Verification items for the finished model (mm, model axes). A direction names the side the tool comes from. Coordinates: 2 decimals unless noted, no trailing zeros. Order: outer loops, then holes, each group sorted by start corner. A loop starts at its lowest first (then second) coordinate and runs counter-clockwise, first axis right, second up. Notation, with made-up numbers: M 6.25,42 L 44.25,42 A10 ccw 44.25,57 Z; hole C 48,60.25 d11. An arc over 180 degrees is marked long. Return JSON: item names as keys, results as strings. Group by question number.
Q1. Thickness scan on probe 1 along Z at (x, y) = (-0.95, 0); probe 2 along X at (y, z) = (0.15, 30); probe 3 along Y at (x, z) = (-0.95, 3). Record the ranges inside material, lowest first.
Q2. Section check C-C, the plane z = 3. Enter the section's corners in (x, y), then the cut area to 3 significant figures.
Q3. Section check A-A, the plane y = 0. Enter the section's corners in (x, z), then the cut area to 4 significant figures.
Q4. Mould release check, pull along X, two halves, no side actions. Record for faces 3 (the face through (-0.5, 0, 5)), 4 (the face through (-2, 0, 20)), 5 (the face through (1.4, 0, 0.4)): pulls with the +X half, pulls with the -X half, needs draft (parallel to the pull), parting line crosses it, or undercut.
Q5. Go/stop test with flat-tipped pins: pin 1 Ø0.8 at (x, y) = (0, 0.5) entering from -Z; pin 2 Ø1.8 at (y, z) = (0, 3) entering from +X; pin 3 Ø1.2 at (y, z) = (-0.5, 2.5) entering from -X. Record where each tip stops, or that it passes through.
Q6. Section check D-D, the plane z = 10. Enter the section's corners in (x, y).
Q7. Section check B-B, the plane x = 0. Enter the section's corners in (y, z), then the cut area to 3 significant figures.
Q8. Access from +Z, -Z, +X, -X, +Y, -Y to the whole of each face (thin tool, end or side, straight path). Record for faces 1 (the face through (0.5, 0, 5)), 2 (the face through (-1, 0, 2)).
from build123d import *

# Parameters (mm, degrees)
SKETCH_1_R                 = 2
EXTRUDE_338_DEPTH          = 40
CHAMFER_1_SIZE             = 1
CUT_EXTRUDE_518_DEPTH      = 41.099875312
CUT_EXTRUDE_518_DEPTH_BACK = 41.099875312
SKETCH_2_W                 = 1
SKETCH_2_H                 = 7.5
CUT_EXTRUDE_2_DEPTH        = 41.099875312
CUT_EXTRUDE_2_DEPTH_BACK   = 41.099875312
SKETCH_3_R                 = 1


with BuildPart() as part:
    # Эскиз1 → Extrude 338 (new body)
    with BuildSketch(Plane.XY):
        Circle(SKETCH_1_R)
    extrude(amount=EXTRUDE_338_DEPTH)

    # Фаска1
    chamfer_1_edges = [part.edges().sort_by_distance(p)[0] for p in [
        (-2, 0, 0),
        (-2, 0, 40),
    ]]
    chamfer(chamfer_1_edges, length=CHAMFER_1_SIZE)

    # Эскиз2 → Cut-Extrude 518 (cut, two sides: drawn at the far end of the back side and taken through both)
    with BuildSketch(Plane(origin=(0, 0, 0), x_dir=(1, 0, 0), z_dir=(0, 1, 0)).offset(-CUT_EXTRUDE_518_DEPTH_BACK)):
        with Locations((0, -3.75)):
            Rectangle(SKETCH_2_W, SKETCH_2_H)
    extrude(amount=CUT_EXTRUDE_518_DEPTH + CUT_EXTRUDE_518_DEPTH_BACK, mode=Mode.SUBTRACT)

    # Эскиз3 → Вырез-Вытянуть2 (cut, two sides: drawn at the far end of the back side and taken through both)
    with BuildSketch(Plane(origin=(0, 0, 0), x_dir=(0, 0, -1), z_dir=(1, 0, 0)).offset(-CUT_EXTRUDE_2_DEPTH_BACK)):
        with Locations((-3, 0)):
            Circle(SKETCH_3_R)
    extrude(amount=CUT_EXTRUDE_2_DEPTH + CUT_EXTRUDE_2_DEPTH_BACK, mode=Mode.SUBTRACT)


solid = part.part
Numbers:
{
 "1": {"probe 1": "z = 0 to 2, 4 to 40", "probe 2": "x = -1.99 to 1.99", "probe 3": "y = -1.76 to -1, 1 to 1.76"},
 "2": {"outline": "M -1.73,-1 A2 ccw -0.5,-1.94 L -0.5,-1 Z; M -1.73,1 L -0.5,1 L -0.5,1.94 A2 ccw Z; M 0.5,-1.94 A2 ccw 1.73,-1 L 0.5,-1 Z; M 0.5,1 L 1.73,1 A2 ccw 0.5,1.94 Z", "area": "2.96 mm2"},
 "3": {"outline": "M -2,1 L -1,0 L -0.5,0 L -0.5,2 L -2,2 Z; M -2,4 L -0.5,4 L -0.5,7.5 L 0.5,7.5 L 0.5,4 L 2,4 L 2,39 L 1,40 L -1,40 L -2,39 Z; M 0.5,0 L 1,0 L 2,1 L 2,2 L 0.5,2 Z", "area": "144.5 mm2"},
 "4": {"face 3": "undercut", "face 4": "parting line crosses it", "face 5": "pulls with the +X half"},
 "5": {"pin 1": "stops at z = 7.5", "pin 2": "passes through", "pin 3": "stops at x = -1.99"},
 "6": {"outline": "C 0,0 d4"},
 "7": {"outline": "M -2,7.5 L 2,7.5 L 2,39 L 1,40 L -1,40 L -2,39 Z", "area": "129 mm2"},
 "8": {"face 1": "-Z, +Y, -Y", "face 2": "+X, -X"}
}
